Part model, mm, in its own coordinate system. Coordinates: 2 decimals unless noted, no trailing zeros. Write each loop counter-clockwise with the first axis right and the second up, starting at its lowest first coordinate (ties: lowest second). Pieces come first, ordered by that corner, then holes. Notation, with made-up numbers: (-15.5, 26) - (31.5, 26) arc R33 cw to (31.5, 64) - close; hole circle Ø6 at (82, -11). An arc over 180 degrees is marked (long way). Use one line per item in the form item = value. Start each with the question number.
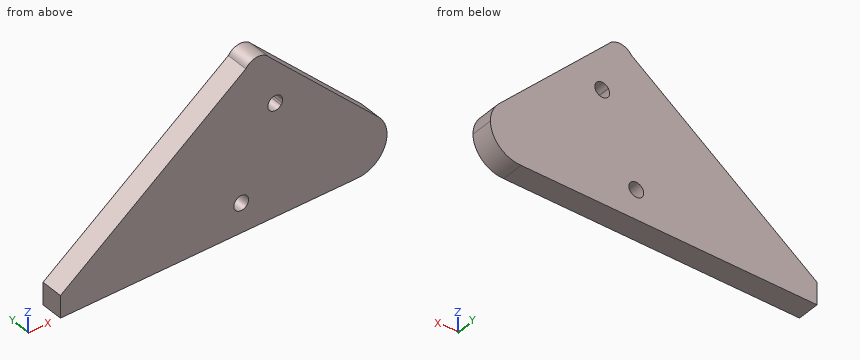
from build123d import *

# Parameters (mm, degrees)
F1_DEPTH = 19.05


with BuildPart() as f1:
    # F0 (on Front) → F1 (new body)
    with BuildSketch(Plane.XZ):
        with BuildLine():
            Line((113.547035, 18.312154), (20.207565, 111.83846))
            ThreePointArc((20.207565, 111.83846), (21.952168, 108.413993), (22.553312, 104.618043))
            ThreePointArc((22.553312, 104.618043), (6.747525, 92.847809), (0, 111.363538))
            Line((0, 111.363538), (-159.037881, -6.186257))
            Line((-159.037881, -6.186257), (-159.037881, -25.236257))
            Line((-159.037881, -25.236257), (94.955072, -25.236257))
            ThreePointArc((94.955072, -25.236257), (72.452371, 10.113642), (113.547035, 18.312154))
        make_face()
        with BuildLine():
            ThreePointArc((2.424053, 0.002768), (2.42405, -0.003481), (2.424041, -0.00973))
            ThreePointArc((2.424041, -0.00973), (-10.275944, 0.009017), (2.424053, 0.002768))
        make_face(mode=Mode.SUBTRACT)
        with BuildLine():
            ThreePointArc((20.120882, 74.508201), (27.224866, 76.854369), (31.632038, 70.808881))
            ThreePointArc((31.632038, 70.808881), (31.506941, 69.554654), (31.136578, 68.349845))
            ThreePointArc((31.136578, 68.349845), (30.759822, 67.596968), (30.286779, 66.900549))
            ThreePointArc((30.286779, 66.900549), (21.64081, 65.606578), (19.896414, 74.173038))
            ThreePointArc((19.896414, 74.173038), (20.005986, 74.342402), (20.120882, 74.508201))
        make_face(mode=Mode.SUBTRACT)
        with BuildLine():
            Line((114.011193, 17.847066), (113.547035, 18.312154))
            ThreePointArc((113.547035, 18.312154), (72.452371, 10.113642), (94.955072, -25.236257))
            ThreePointArc((94.955072, -25.236257), (113.459019, -18.111528), (121.200292, 0.143075))
            ThreePointArc((121.200292, 0.143075), (119.334471, 9.697059), (114.011193, 17.847066))
        make_face()
        with BuildLine():
            ThreePointArc((22.553312, 104.618043), (21.952168, 108.413993), (20.207565, 111.83846))
            ThreePointArc((20.207565, 111.83846), (9.979243, 116.900066), (0, 111.363538))
            ThreePointArc((0, 111.363538), (6.747525, 92.847809), (22.553312, 104.618043))
        make_face()
    extrude(amount=F1_DEPTH)


solid = f1.part
Q1. Slice it at C-C (z = 80.5). List the corners of the cut face in (x, y).
Q2. Pin check, flat tips, straight feed: P1, Ø8, axis at x = 31.5, y = -4.5, coming from the +Z side; P2, Ø4, axis at x = -65, y = -16, coming from the +Z side; P3, Ø8, axis at y = -2.5, z = 39.5, coming from the -X side. Stop position of each tip, or through.
Q3. Slice it at A-A (y = -11.75). Count the separate pieces of the cut face and the enclosed holes in it, plus the area to 3 significant figures.
Q4. Slice it at B-B (x = 26.5). List the corners of the cut face in (y, z).
Q5. Drill centre lines: probe 1 along X at (y, z) = (-0.75, 66); probe 2 along Z at (x, y) = (-90, -12.5); probe 3 along X at (y, z) = (-10, 95.5). Where is each one in solid material? Low to high.
Q6. Slice it at D-D (x = -28). List the corners of the cut face in (y, z), plus the area to 3 significant figures.
Solution:
q1.outline = (-41.76, -19.05) - (51.48, -19.05) - (51.48, 0) - (-41.76, 0) - close
q2.P1 = 104.53
q2.P2 = 64.8
q2.P3 = -102.64
q3.separate_pieces = 1
q3.enclosed_holes = 2
q3.area = 23,500 mm2
q4.outline = (-19.05, -25.24) - (0, -25.24) - (0, 64.58) - (-19.05, 64.58) - close; (-19.05, 77.04) - (0, 77.04) - (0, 105.53) - (-19.05, 105.53) - close
q5.probe_1 = -61.37 to 21.14, 29.43 to 65.95
q5.probe_2 = -25.24 to 44.84
q5.probe_3 = -21.46 to 36.51
q6.outline = (-19.05, -25.24) - (0, -25.24) - (0, 90.67) - (-19.05, 90.67) - close
q6.area = 2,210 mm2
